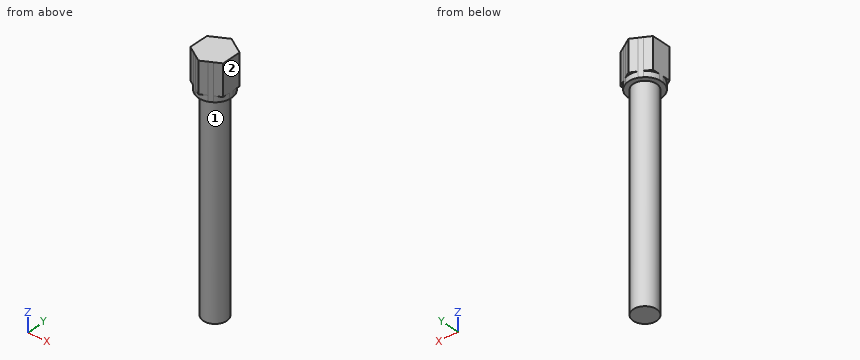
```python
from build123d import *

# Parameters (mm, degrees)
F0_R     = 6
F1_DEPTH = 16
F2_DEPTH = 3
F3_DEPTH = 110


with BuildPart() as f1:
    # F0 (on Top) → F1 (new body)
    with BuildSketch(Plane.XY):
        with BuildLine():
            Line((8.425, -1.1266654339), (8.425, 1.1266654339))
            ThreePointArc((8.425, 1.1266654339), (7.3612159322, 4.25), (5.1882208873, 6.7329313099))
            Line((5.1882208873, 6.7329313099), (3.2367791127, 7.8595967438))
            ThreePointArc((3.2367791127, 7.8595967438), (0, 8.5), (-3.2367791127, 7.8595967438))
            Line((-3.2367791127, 7.8595967438), (-5.1882208873, 6.7329313099))
            ThreePointArc((-5.1882208873, 6.7329313099), (-7.3612159322, 4.25), (-8.425, 1.1266654339))
            Line((-8.425, 1.1266654339), (-8.425, -1.1266654339))
            ThreePointArc((-8.425, -1.1266654339), (-7.3612159322, -4.25), (-5.1882208873, -6.7329313099))
            Line((-5.1882208873, -6.7329313099), (-3.2367791127, -7.8595967438))
            ThreePointArc((-3.2367791127, -7.8595967438), (0, -8.5), (3.2367791127, -7.8595967438))
            Line((3.2367791127, -7.8595967438), (5.1882208873, -6.7329313099))
            ThreePointArc((5.1882208873, -6.7329313099), (7.3612159322, -4.25), (8.425, -1.1266654339))
        make_face()
        Circle(F0_R, mode=Mode.SUBTRACT)
        with BuildLine():
            ThreePointArc((-8.425, 1.1266654339), (-7.3612159322, 4.25), (-5.1882208873, 6.7329313099))
            Line((-5.1882208873, 6.7329313099), (-8.425, 4.8641760179))
            Line((-8.425, 4.8641760179), (-8.425, 1.1266654339))
        make_face()
        with BuildLine():
            Line((-8.425, -4.8641760179), (-5.1882208873, -6.7329313099))
            ThreePointArc((-5.1882208873, -6.7329313099), (-7.3612159322, -4.25), (-8.425, -1.1266654339))
            Line((-8.425, -1.1266654339), (-8.425, -4.8641760179))
        make_face()
        with BuildLine():
            Line((0, -9.7283520358), (3.2367791127, -7.8595967438))
            ThreePointArc((3.2367791127, -7.8595967438), (0, -8.5), (-3.2367791127, -7.8595967438))
            Line((-3.2367791127, -7.8595967438), (0, -9.7283520358))
        make_face()
        with BuildLine():
            Line((8.425, -4.8641760179), (8.425, -1.1266654339))
            ThreePointArc((8.425, -1.1266654339), (7.3612159322, -4.25), (5.1882208873, -6.7329313099))
            Line((5.1882208873, -6.7329313099), (8.425, -4.8641760179))
        make_face()
        with BuildLine():
            ThreePointArc((5.1882208873, 6.7329313099), (7.3612159322, 4.25), (8.425, 1.1266654339))
            Line((8.425, 1.1266654339), (8.425, 4.8641760179))
            Line((8.425, 4.8641760179), (5.1882208873, 6.7329313099))
        make_face()
        with BuildLine():
            ThreePointArc((-3.2367791127, 7.8595967438), (0, 8.5), (3.2367791127, 7.8595967438))
            Line((3.2367791127, 7.8595967438), (0, 9.7283520358))
            Line((0, 9.7283520358), (-3.2367791127, 7.8595967438))
        make_face()
        Circle(F0_R)
    extrude(amount=F1_DEPTH)

    # F0 (on Top) → F2 (join)
    with BuildSketch(Plane.XY):
        with BuildLine():
            Line((8.425, -1.1266654339), (8.425, 1.1266654339))
            ThreePointArc((8.425, 1.1266654339), (7.3612159322, 4.25), (5.1882208873, 6.7329313099))
            Line((5.1882208873, 6.7329313099), (3.2367791127, 7.8595967438))
            ThreePointArc((3.2367791127, 7.8595967438), (0, 8.5), (-3.2367791127, 7.8595967438))
            Line((-3.2367791127, 7.8595967438), (-5.1882208873, 6.7329313099))
            ThreePointArc((-5.1882208873, 6.7329313099), (-7.3612159322, 4.25), (-8.425, 1.1266654339))
            Line((-8.425, 1.1266654339), (-8.425, -1.1266654339))
            ThreePointArc((-8.425, -1.1266654339), (-7.3612159322, -4.25), (-5.1882208873, -6.7329313099))
            Line((-5.1882208873, -6.7329313099), (-3.2367791127, -7.8595967438))
            ThreePointArc((-3.2367791127, -7.8595967438), (0, -8.5), (3.2367791127, -7.8595967438))
            Line((3.2367791127, -7.8595967438), (5.1882208873, -6.7329313099))
            ThreePointArc((5.1882208873, -6.7329313099), (7.3612159322, -4.25), (8.425, -1.1266654339))
        make_face()
        Circle(F0_R, mode=Mode.SUBTRACT)
        Circle(F0_R)
    extrude(amount=-F2_DEPTH)

    # F0 (on Top) → F3 (join)
    with BuildSketch(Plane.XY):
        Circle(F0_R)
    extrude(amount=-F3_DEPTH)


solid = f1.part
```
Here's how the part is built. I have some questions about the finished solid (model axes, mm). Face numbers are marked on the shaded views. A direction names the side the tool comes from. Coordinates: 2 decimals unless noted, no trailing zeros. Write each loop counter-clockwise with the first axis right and the second up, starting at its lowest first coordinate (ties: lowest second). Pieces come first, ordered by that corner, then holes. Notation, with made-up numbers: M 48.25,33.5 L 74.25,33.5 A32 cw 74.25,61.5 Z; hole C 15,48.5 d4. An arc over 180 degrees is marked long. Answer as CSV lines item,"result". Start each with the question number.
Q1. Will these pins go through, and if not, where does the flat tip stop? pin 1 Ø1 at (x, z) = (-2.5, -7.5) entering from +Y; pin 2 Ø3 at (x, z) = (2.5, -22.5) entering from -Y; pin 3 Ø2.5 at (x, y) = (-6, 4) entering from -Z; pin 4 Ø2.5 at (x, y) = (7.5, 3) entering from -Z.
Q2. Suppose I cut it at B-B, the plane z = -82.5. List the corners of the cut face in (x, y) for me.
Q3. I need wall thicknesses on probe 1 along Z at (x, y) = (-2.25, 8); probe 2 along Y at (x, z) = (-3.5, -18.5); probe 3 along Y at (x, z) = (-5, -95.5). Which ranges of each line are inside material? Lowest first, please. Write a range as [from, to].
Q4. Suppose I cut it at A-A, the plane y = 0. List the corners of the cut face in (x, z) for me (3 decimals).
Q5. For the marked faces 1 and 2, which set-ups out of +Z, -Z, +X, -X, +Y, -Y let a thin tool reach every point of the face, with its end or its side?
Entries:
1,pin 1,"stops at y = 5.66"
1,pin 2,"stops at y = -5.92"
1,pin 3,"stops at z = -110"
1,pin 4,"stops at z = -3"
2,outline,"C 0,0 d12"
3,probe 1,"z = [-3, 16]"
3,probe 2,"y = [-4.87, 4.87]"
3,probe 3,"y = [-3.32, 3.32]"
4,outline,"M -8.425,-3 L -6,-3 L -6,-110 L 6,-110 L 6,-3 L 8.425,-3 L 8.425,16 L -8.425,16 Z"
5,face 1,"-Z"
5,face 2,"+Z, -Z, +X, +Y, -Y"
